Design review of the part built by this model. Coordinates are the model's own, in mm. Give positions to 0.01 mm unless a question says otherwise; leave off trailing zeros. Write each loop counter-clockwise with the first axis right and the second up, starting at its lowest first coordinate (ties: lowest second). Pieces come first, ordered by that corner, then holes. Notation, with made-up numbers: M 23.25,-9 L 71.25,-9 A10 cw 71.25,-1 Z; hole C -21.75,19 d8. An arc over 180 degrees is marked long. Write each question's results on one line, items separated by ' | '. Start each with the question number.
from build123d import *

# Parameters (mm, degrees)
SKETCH1_R             = 4
BOSS_EXTRUDE1_DEPTH   = 25
CHAMFER1_SIZE         = 1
M5_TAPPED_HOLE1_D     = 4.2
M5_TAPPED_HOLE1_DEPTH = 6
M5_TAPPED_HOLE1_TIP   = 1.2618073


with BuildPart() as part:
    # Sketch1 → Boss-Extrude1 (new body)
    with BuildSketch(Plane(origin=(0, 0, 0), x_dir=(1, 0, 0), z_dir=(0, 1, 0))):
        Circle(SKETCH1_R)
    extrude(amount=BOSS_EXTRUDE1_DEPTH)

    # Chamfer1
    chamfer1_edges = [part.edges().sort_by_distance(p)[0] for p in [
        (-4, 25, 0),
    ]]
    chamfer(chamfer1_edges, length=CHAMFER1_SIZE)

    # M5 Tapped Hole1
    with Locations(Plane.XZ):
        with Locations((0, 0)):
            Hole(M5_TAPPED_HOLE1_D / 2, depth=M5_TAPPED_HOLE1_DEPTH)
            with Locations((0, 0, -(M5_TAPPED_HOLE1_DEPTH + M5_TAPPED_HOLE1_TIP / 2))):  # 118° drill point
                Cone(0, M5_TAPPED_HOLE1_D / 2, M5_TAPPED_HOLE1_TIP, mode=Mode.SUBTRACT)


solid = part.part
Q1. Wall thickness on line 1 along Z through (x, y) = (0, 4); line 2 along X through (y, z) = (2.25, -0.75): over which ranges is each line inside the solid? List them lowest first. Write a range as from..to.
Q2. We need section A-A on y = 5. Write out the cut boundary in (x, z), and give its area (3 significant figures).
Q3. The part is to be moulded in two halves that separate along Z. For faces 1 (the cylindrical face through (-2.003, 3.042, 0.631)), 2 (the flat face through (2, 0, 2)), 3 (the cylindrical face through (-0.867, 11.832, 3.905)), say which applies: pulls with the +Z half, pulls with the -Z half, needs draft (parallel to the pull), parting line crosses it, or undercut.
Q4. We need section B-B on y = 14.25. Write out the cut boundary in (x, z), and give its area (3 significant figures).
Q5. For pin 1 Ø3 at (x, y) = (-2, 7) entering from -Z; pin 2 Ø2 at (x, y) = (2, 16) entering from -Z; pin 3 Ø4 at (x, z) = (0, 0) entering from -Y, all flat-tipped, find the tip position at first contact; note any pin that passes through.
Answer sheet:
1) line 1: -4..-2.1, 2.1..4 | line 2: -3.93..-1.96, 1.96..3.93
2) outline: C 0,0 d8; hole C 0,0 d4.2 | area: 36.4 mm^2
3) face 1: undercut | face 2: needs draft | face 3: parting line crosses it
4) outline: C 0,0 d8 | area: 50.3 mm^2
5) pin 1: z = -3.97 | pin 2: z = -3.87 | pin 3: y = 6.06
